The listing builds one solid part. Answer for the finished solid, in the listing's coordinates (mm). A direction names the side the tool comes from. Coordinates: 2 decimals unless noted, no trailing zeros. Order: outer loops, then holes, each group sorted by start corner. A loop starts at its lowest first (then second) coordinate and runs counter-clockwise, first axis right, second up. Notation, with made-up numbers: M 33,-6.75 L 60,-6.75 A32 ccw 60,22.25 Z; hole C 21.5,-27 d10. An arc over 180 degrees is marked long. One line per item, written item: value. Start each with the question number.
Q1. The part is cut by section C-C on x = -21. Give the vertices of the cut face in (y, z), then the cut area to 3 significant figures.
Q2. The part is cut by section D-D on z = 13.5. Give the vertices of the cut face in (x, y), then the cut area to 3 significant figures.
Q3. Determine the mould class of faces 1 (the cylindrical face through (15.148, -46.047, 12.325)), 2 (the cylindrical face through (-20.377, -40.256, 12.325)), 3 (the flat face through (48.098, 15, 12)), 4 (the flat face through (-33.15, -42.14, 12.32)) for opening direction X: pulls with the +X half, pulls with the -X half, needs draft (parallel to the pull), parting line crosses it, or undercut.
Q4. Straight lines are drawn through the part: line 1 along X through (y, z) = (14.5, 18.75); line 2 along Y through (x, z) = (-2, 10.25); line 3 along Y through (x, z) = (15.5, 7.5). For each, find the intervals that lie inside material, in ascending order. Write a range as [from, to].
Q5. Each of these flat-tipped pins is pushed along its axis until it touches: pin 1 Ø1.5 at (x, z) = (-37, 13.5) entering from -Y; pin 2 Ø10 at (x, z) = (-43.5, 10.5) entering from +Y; pin 3 Ø3 at (y, z) = (-34, 14.5) entering from -X; pin 4 Ø6.5 at (x, y) = (-20.38, 56.74) entering from -Z. Where does it stop, or does it pass through?
Q6. The part is cut by section A-A on y = 22. Give the vertices of the cut face in (x, z), then the cut area to 3 significant figures.
Q7. For faces 5 (the flat face through (-42.8, -24.79, 12.32)), 6 (the flat face through (-42.321, -6.613, 12.325)), determine the directions among +Z, -Z, +X, -X, +Y, -Y from which every point of the face is accessible in a straight line to the end or side of a thin tool.
Q8. The part is cut by section B-B on x = -2.5. Give the vertices of the cut face in (y, z).
```python
from build123d import *

# Parameters (mm, degrees)
F0_R     = 3.9401235554
F0_R_2   = 3.7179654295
F0_R_3   = 2.4821275962
F0_R_4   = 3.0762994678
F1_DEPTH = 25


with BuildPart() as f1:
    # F0 (on Top) → F1 (new body)
    with BuildSketch(Plane.XY):
        Polygon((25.9239133447, 61.9565248489), (-29.1847828776, 61.9565248489), (-37.0108708739, 50.2173937857), (-24.6630428207, 50.2173937857), (24.6195662767, 50.2173937857), (36.0326059163, 50.2173937857), align=None)
        with Locations((-20.3804355115, 56.7391328514)):
            Circle(F0_R, mode=Mode.SUBTRACT)
        with Locations((17.7717413753, 57.7173940837)):
            Circle(F0_R_2, mode=Mode.SUBTRACT)
        Polygon((-29.1847828776, 45.0000013742), (-37.0108708739, 50.2173937857), (-53.9673939347, 30.6521747261), (-46.3995258629, 25.1368362456), align=None)
        Polygon((-24.6630428207, 50.2173937857), (-37.0108708739, 50.2173937857), (-29.1847828776, 45.0000013742), align=None)
        Polygon((28.6701515291, 44.7763084559), (36.0326059163, 50.2173937857), (24.6195662767, 50.2173937857), align=None)
        Polygon((48.0978302658, 30.6521747261), (36.0326059163, 50.2173937857), (28.6701515291, 44.7763084559), (39.184783137, 30.6521747261), (39.184783137, 0), (33.0978259444, -9.1304350644), (21.3586967438, -35.8695648611), (30.815217644, -35.8695648611), (41.9021770358, -13.0434790626), (48.0978302658, 0), align=None)
        Polygon((-46.3995258629, 25.1368362456), (-53.9673939347, 30.6521747261), (-53.9673939347, 0), (-48.4239161015, -14.0217393637), (-37.0108708739, -35.8695648611), (-26.4319663345, -35.8695648611), (-38.3560431547, -13.0434790626), (-46.3995258629, 0), align=None)
        Polygon((-26.4319663345, -35.8695648611), (-37.0108708739, -35.8695648611), (-29.1847828776, -48.5869571567), (27.8804339468, -48.5869571567), (30.815217644, -35.8695648611), (21.3586967438, -35.8695648611), align=None)
        with Locations((-20.0543478131, -42.7173897624)):
            Circle(F0_R_3, mode=Mode.SUBTRACT)
        with Locations((15.8152170479, -43.0434793234)):
            Circle(F0_R_4, mode=Mode.SUBTRACT)
    extrude(amount=F1_DEPTH)


solid = f1.part
```
Output:
1. outline: M -48.59,0 L -45.01,0 L -45.01,25 L -48.59,25 Z; M -40.42,0 L -35.87,0 L -35.87,25 L -40.42,25 Z; M 50.22,0 L 52.85,0 L 52.85,25 L 50.22,25 Z; M 60.63,0 L 61.96,0 L 61.96,25 L 60.63,25 Z
1. area: 302 mm^2
2. outline: M -53.97,0 L -48.42,-14.02 L -37.01,-35.87 L -29.18,-48.59 L 27.88,-48.59 L 30.82,-35.87 L 41.9,-13.04 L 48.1,0 L 48.1,30.65 L 36.03,50.22 L 25.92,61.96 L -29.18,61.96 L -37.01,50.22 L -53.97,30.65 Z; hole M -46.4,0 L -38.36,-13.04 L -26.43,-35.87 L 21.36,-35.87 L 33.1,-9.13 L 39.18,0 L 39.18,30.65 L 24.62,50.22 L -24.66,50.22 L -46.4,25.14 Z; hole C -20.38,56.74 d7.88; hole C -20.05,-42.72 d4.96; hole C 15.82,-43.04 d6.15; hole C 17.77,57.72 d7.44
2. area: 3,080 mm^2
3. face 1: undercut
3. face 2: undercut
3. face 3: pulls with the +X half
3. face 4: pulls with the -X half
4. line 1: x = [-53.97, -46.4], [39.18, 48.1]
4. line 2: y = [-48.59, -35.87], [50.22, 61.96]
4. line 3: y = [-48.59, -46.1], [-39.98, -35.87], [50.22, 54.77], [60.66, 61.96]
5. pin 1: stops at y = -37.11
5. pin 2: stops at y = 48.5
5. pin 3: stops at x = -38.77
5. pin 4: passes through
6. outline: M -53.97,0 L -46.4,0 L -46.4,25 L -53.97,25 Z; M 39.18,0 L 48.1,0 L 48.1,25 L 39.18,25 Z
6. area: 412 mm^2
7. face 5: +Z, -Z, -X, -Y
7. face 6: +Z, -Z
8. outline: M -48.59,0 L -35.87,0 L -35.87,25 L -48.59,25 Z; M 50.22,0 L 61.96,0 L 61.96,25 L 50.22,25 Z
